Could you check a few things on this drawing? It's one solid part, dimensions in mm from its lowest x, y, z. A direction names the side the tool comes from. Round coordinates to 2 decimals unless told otherwise and drop trailing zeros. Loops run counter-clockwise (first coordinate to the right, second up) from the corner with the lowest first, then second, coordinate; pieces in that order, holes last. Notation, with made-up numbers: (80.25, 20) -> (94.25, 20) arc R19 ccw to (94.25, 38) -> close; hole circle Ø7 at (-2.75, 24). An arc over 180 degrees is marked (long way). Put each result on its own line as item: value. Start each with the question number.
1. Imagine slicing it at C-C, the plane z = 36.5. Please give me the cut outline in (x, y).
2. I'm going to push a flat-ended pin straight in: P1, Ø5, axis at x = 6, y = 2.5, coming from the -Z side. Where does the tip first touch, or does it pass through?
3. Which directions (+Z, -Z, +X, -X, +Y, -Y) give clear straight access to the entire face, cutting with the end or side of a thin tool? Please do the marked faces 1 and 2.
4. I need wall thicknesses on line 1 (Y direction, x = 2.25, z = 27); line 2 (Z direction, x = 7, y = 4). Which ranges of each line are inside material? Lowest first, please. Write a range as [from, to].
5. Imagine slicing it at A-A, the plane x = 6. Please give me the cut outline in (y, z).
6. Imagine slicing it at B-B, the plane y = 1.5. Please give me the cut outline in (x, z).
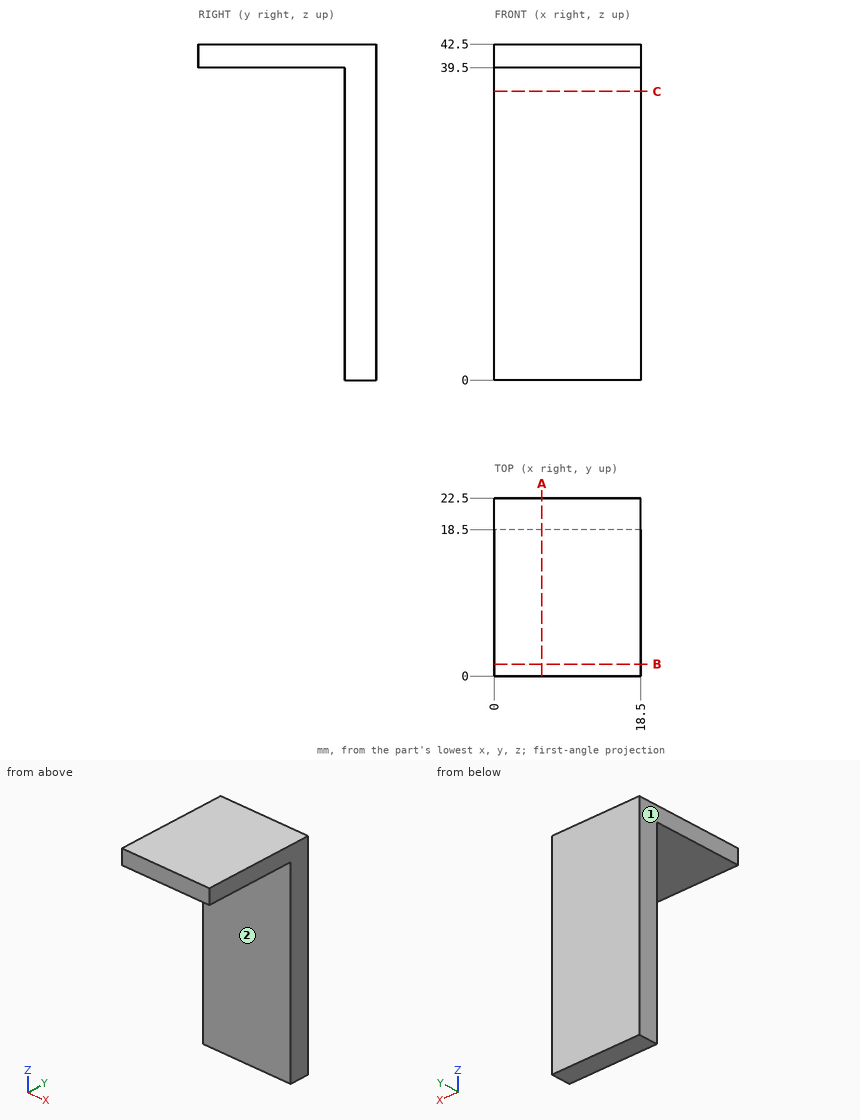
Entries:
1. outline: (0, 18.5) -> (18.5, 18.5) -> (18.5, 22.5) -> (0, 22.5) -> close
2. P1: z = 39.5
3. face 1: +Z, -Z, -X, +Y, -Y
3. face 2: -Z, +X, -X, -Y
4. line 1: [18.5, 22.5]
4. line 2: [39.5, 42.5]
5. outline: (0, 39.5) -> (18.5, 39.5) -> (18.5, 0) -> (22.5, 0) -> (22.5, 42.5) -> (0, 42.5) -> close
6. outline: (0, 39.5) -> (18.5, 39.5) -> (18.5, 42.5) -> (0, 42.5) -> close
